Autodesk Inventor part; units mm, degrees
ref_plane "YZ Plane" through (0, 0, 0) normal (1, 0, 0) x (0, 1, 0)
ref_plane "XZ Plane" through (0, 0, 0) normal (0, 1, 0) x (-1, 0, 0)
ref_plane "XY Plane" through (0, 0, 0) normal (0, 0, 1) x (1, 0, 0)
sketch "Sketch1" plane through (0, 0, 0) normal (0, 0, 1) x (1, 0, 0)
  arc A0 (0, -4.125) -> (-4.0608, 0.7248) centre (0, 0) ccw
  line L0 (0, -4.125) -> (-4.0608, 0.7248)
  arc A1 (-0.4919, -5.3424) -> (-5.3588, 0.2578) centre (0, 0) ccw
  line L1 (0, -4.125) -> (-0.4919, -5.3424)
  line L2 (0, -4.125) -> (1.313, -4.125) construction
  line L3 (-4.0608, 0.7248) -> (-5.3588, 0.2578)
  dimension "d0" = 8.25
  dimension "d1" = 10.73
  dimension "d2" = 112
extrude "Extrusion1" add sketch "Sketch1" along normal blind 19 contours A0 L3 A1 L1
sketch "Sketch2" plane through (0, 0, 19) normal (0, 0, 1) x (1, 0, 0)
  arc A0 (-0.4919, -5.3424) -> (-5.3588, 0.2578) centre (0, 0) ccw
  line L0 (0, 5.365) -> (5.365, 0) construction
  line L1 (3.7936, 3.7936) -> (0, 5.365) construction
  line L2 (3.7936, 3.7936) -> (5.365, 0) construction
  line L3 (3.7936, 3.7936) -> (5.5269, 2.0604)
  line L4 (5.5269, 2.0604) -> (35.5269, 32.0604)
  line L5 (35.5269, 32.0604) -> (33.7936, 33.7936)
  line L6 (33.7936, 33.7936) -> (3.7936, 3.7936)
  line L7 (1.9965, 5.5907) -> (31.9965, 35.5907)
  line L8 (31.9965, 35.5907) -> (33.7936, 33.7936)
  line L9 (1.9965, 5.5907) -> (3.7936, 3.7936)
  line L10 (1.9965, 5.5907) -> (5.5269, 2.0604)
  line L11 (5.5269, 2.0604) -> (4.7391, 1.2726)
  line L12 (4.7391, 1.2726) -> (1.2088, 4.8029)
  line L13 (1.2088, 4.8029) -> (1.9965, 5.5907)
  line L14 (-3.7936, 3.7936) -> (-5.365, 0) construction
  line L15 (-3.7936, 3.7936) -> (-2.0604, 5.5269)
  line L16 (-2.0604, 5.5269) -> (-32.0604, 35.5269)
  line L17 (-32.0604, 35.5269) -> (-33.7936, 33.7936)
  line L18 (-33.7936, 33.7936) -> (-3.7936, 3.7936)
  line L19 (-5.5907, 1.9965) -> (-35.5907, 31.9965)
  line L20 (-35.5907, 31.9965) -> (-33.7936, 33.7936)
  line L21 (-5.5907, 1.9965) -> (-3.7936, 3.7936)
  line L22 (-5.5907, 1.9965) -> (-2.0604, 5.5269)
  line L23 (-2.0604, 5.5269) -> (-1.2726, 4.7391)
  line L24 (-1.2726, 4.7391) -> (-4.8029, 1.2088)
  line L25 (-4.8029, 1.2088) -> (-5.5907, 1.9965)
  line L26 (-3.7936, -3.7936) -> (0, -5.365) construction
  line L27 (-3.7936, -3.7936) -> (-5.5269, -2.0604)
  line L28 (-5.5269, -2.0604) -> (-35.5269, -32.0604)
  line L29 (-35.5269, -32.0604) -> (-33.7936, -33.7936)
  line L30 (-33.7936, -33.7936) -> (-3.7936, -3.7936)
  line L31 (-1.9965, -5.5907) -> (-31.9965, -35.5907)
  line L32 (-31.9965, -35.5907) -> (-33.7936, -33.7936)
  line L33 (-1.9965, -5.5907) -> (-3.7936, -3.7936)
  line L34 (-1.9965, -5.5907) -> (-5.5269, -2.0604)
  line L35 (-5.5269, -2.0604) -> (-4.7391, -1.2726)
  line L36 (-4.7391, -1.2726) -> (-1.2088, -4.8029)
  line L37 (-1.2088, -4.8029) -> (-1.9965, -5.5907)
  line L38 (3.7936, -3.7936) -> (5.365, 0) construction
  line L39 (3.7936, -3.7936) -> (2.0604, -5.5269)
  line L40 (2.0604, -5.5269) -> (32.0604, -35.5269)
  line L41 (32.0604, -35.5269) -> (33.7936, -33.7936)
  line L42 (33.7936, -33.7936) -> (3.7936, -3.7936)
  line L43 (5.5907, -1.9965) -> (35.5907, -31.9965)
  line L44 (35.5907, -31.9965) -> (33.7936, -33.7936)
  line L45 (5.5907, -1.9965) -> (3.7936, -3.7936)
  line L46 (5.5907, -1.9965) -> (2.0604, -5.5269)
  line L47 (2.0604, -5.5269) -> (1.2726, -4.7391)
  line L48 (1.2726, -4.7391) -> (4.8029, -1.2088)
  line L49 (4.8029, -1.2088) -> (5.5907, -1.9965)
  dimension "d5" = 30
  dimension "d6" = 30
  dimension "d11" = 360
extrude "Extrusion2" add sketch "Sketch2" against normal blind 2 contours L47 L48 L49 A0 | A0 L39 L47 | L23 L24 L25 A0 | A0 L15 L23 | L11 L12 L13 A0 | A0 L3 L11 | L42 L41 L40 L39 | L45 L43 L44 L42 | A0 L49 L45 | L6 L5 L4 L3 | L9 L7 L8 L6 | A0 L13 L9 | L18 L17 L16 L15 | L21 L19 L20 L18 | A0 L25 L21
sketch "Sketch3" plane through (0, 0, 19) normal (0, 0, 1) x (1, 0, 0)
  circle A0 centre (0, 0) radius 47.75
  circle A1 centre (0, 0) radius 49.75
  dimension "d13" = 95.5
  dimension "d14" = 99.5
extrude "Extrusion3" add sketch "Sketch3" against normal blind 2
sketch "Sketch4" plane through (0, 0, 19) normal (0, 0, 1) x (1, 0, 0)
  line L0 (-57.3156, 53.7161) -> (57.3156, 53.7161)
  line L1 (57.3156, 53.7161) -> (57.3156, -53.7161)
  line L2 (57.3156, -53.7161) -> (-57.3156, -53.7161)
  line L3 (-57.3156, -53.7161) -> (-57.3156, 53.7161)
  line L4 (-57.3156, 53.7161) -> (57.3156, -53.7161) construction
  line L5 (57.3156, 53.7161) -> (-57.3156, -53.7161) construction
  point P0 (0, 0)
extrude "Extrusion4" cut sketch "Sketch4" against normal blind 10
properties part number "GuardTest"
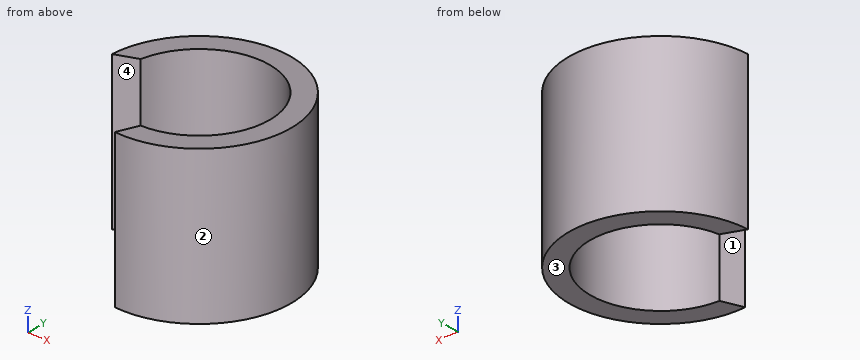
Geometry: final body of the model. Coordinates: model frame, mm. Face numbers are marked on the shaded views. Give positions to 0.01 mm unless a question says otherwise; leave off trailing zeros. Write each loop counter-clockwise with the first axis right and the second up, starting at its lowest first coordinate (ties: lowest second). Pieces come first, ordered by that corner, then holes.
1. Section query A-A, the plane x = 0.5. Return loops of the section in (y, z).
2. Section query D-D, the plane x = 4.5. Return loops of the section in (y, z), then the cut area to 3 significant figures.
3. Draft query along X for the marked faces 1, 2, 3 and 4. Return one class per face: released by +X, released by -X, zero draft, split by the parting line, or undercut.
4. Pin query (flat end, axial travel): P1, Ø2, axis at y = -2, z = 4, coming from the +X side; P2, Ø1.5, axis at x = 1.5, z = 5.5, coming from the -Y side; P3, Ø1.5, axis at x = -1, z = 3.5, coming from the -Y side. Return the tip coordinate at first contact, or that it passes through.
5. Line query: probe 1 along X at (y, z) = (1, 2.5); probe 2 along Y at (x, z) = (2.75, 5); probe 3 along Y at (x, z) = (3, 0.5). Output: solid intervals per line, ascending.
6. Section query C-C, the plane z = 4. Return loops of the section in (x, y) (3 decimals), then the cut area to 3 significant figures.
7. Section query B-B, the plane y = 0.5. Return loops of the section in (x, z), then the cut area to 3 significant figures.
Computed:
1. outline: (-5.34, 0) - (-4.09, 0) - (-4.09, 9) - (-5.34, 9) - close; (4.09, 0) - (5.34, 0) - (5.34, 9) - (4.09, 9) - close
2. outline: (-2.92, 0) - (2.92, 0) - (2.92, 9) - (-2.92, 9) - close
2. area: 52.6 mm2
3. face 1: released by -X
3. face 2: split by the parting line
3. face 3: zero draft
3. face 4: undercut
4. P1: stops at x = 5.27
4. P2: stops at y = -5.31
4. P3: stops at y = -5.36
5. probe 1: x = -5.27 to -4, 4 to 5.27
5. probe 2: y = -4.61 to -3.07, 3.07 to 4.61
5. probe 3: y = -4.45 to -2.83, 2.83 to 4.45
6. outline: (-5.359, 0.258) - (-4.061, 0.725) arc R4.125 cw (long way) to (0, -4.125) - (-0.492, -5.342) arc R5.365 ccw (long way) to start
6. area: 27.4 mm2
7. outline: (-5.34, 0) - (-4.69, 0) - (-4.69, 9) - (-5.34, 9) - close; (4.09, 0) - (5.34, 0) - (5.34, 9) - (4.09, 9) - close
7. area: 17.1 mm2
